Geometry: final body of the model. Coordinates: model frame, mm. A direction names the side the tool comes from. Give positions to 0.01 mm unless a question says otherwise; leave off trailing zeros. Write each loop counter-clockwise with the first axis right and the second up, starting at its lowest first coordinate (ties: lowest second). Pieces come first, ordered by that corner, then holes. Notation, with made-up numbers: M 47,64 L 63,64 A29 cw 63,88 Z; hole C 2.25,55.25 d5. An arc over 180 degrees is marked long. Use one line per item in the form item = value. Start each with the question number.
Item 1: Section query C-C on y = 55.5. Return loops of the section in (x, z).
Item 2: Material intervals for line 1 along Z through (x, y) = (-28.2, 8); line 2 along Y through (x, z) = (-15, -23); line 3 along X through (y, z) = (6, -28) (3 decimals), sorted ascending. Write a range as from..to.
Item 3: Section query D-D on z = -36. Return loops of the section in (x, y), then the cut area to 3 significant figures.
Item 4: Section query B-B on x = -18.5. Return loops of the section in (y, z), then the cut area to 3 significant figures.
Item 5: Contact query for flat-ended pins moving along their axis: P1, Ø5, axis at x = -29.5, y = 60, coming from the -Z side; P2, Ø10, axis at x = -8.5, z = -33, coming from the +Y side; P3, Ø8, axis at x = -24.5, y = 36, coming from the +Z side; P4, Ø3, axis at x = -30, z = -33, coming from the +Y side. Output: stop coordinate, or through.
Item 6: Pull-direction query (Z, two-part tool) for faces 5 (the flat face through (-28, 2, 0)), 6 (the cylindrical face through (-15.19, 25.71, -53.22)), 7 (the cylindrical face through (-24.385, 9.86, -26.999)); classes: released by +Z, released by -Z, zero draft, split by the parting line, or undercut.
Item 7: Section query A-A on y = 11. Return loops of the section in (x, z), then the cut area to 3 significant figures.
Item 8: Access query for faces 1 (the flat face through (-50, 5, -6)), 2 (the flat face through (-6, 5, -7)), 3 (the flat face through (-28, 53, -33)), 4 (the flat face through (-51, 5, -51)). Directions: +Z, -Z, +X, -X, +Y, -Y. A direction counts if a zero-diameter tool reaches every point of the face in a straight line with its end or side. Return the directions, or none.
Autodesk Inventor part; units mm, degrees
ref_plane "YZ Plane" through (0, 0, 0) normal (1, 0, 0) x (0, 1, 0)
ref_plane "XZ Plane" through (0, 0, 0) normal (0, 1, 0) x (-1, 0, 0)
ref_plane "XY Plane" through (0, 0, 0) normal (0, 0, 1) x (1, 0, 0)
sketch "Sketch1" plane through (0, 0, 0) normal (0, 1, 0) x (-1, 0, 0)
  line L0 (0, 0) -> (56.4, 0)
  line L1 (56.4, 0) -> (56.4, -56.4)
  line L2 (56.4, -56.4) -> (0, -56.4)
  line L3 (0, -56.4) -> (0, 0)
  dimension "d0" = 56.4
  dimension "d1" = 56.4
extrude "Extrusion1" add sketch "Sketch1" along normal blind 5
sketch "Sketch2" plane through (0, 5, 0) normal (0, 1, 0) x (1, 0, 0)
  circle A0 centre (-28.2, 28.2) radius 28.2
  line L0 (-56.4, 0) -> (0, 0)
  line L1 (-56.4, 56.4) -> (-56.4, 0)
  dimension "d4" = 56.4
  dimension "d5" = 28.2
  dimension "d6" = 28.2
extrude "Extrusion2" add sketch "Sketch2" along normal blind 42 contours A0
sketch "Sketch3" plane through (-28.2, 47, -28.2) normal (0, 1, 0) x (1, 0, 0)
  arc A0 (0, 28.2) -> (-28.2, 0) centre (0, 0) ccw
  circle A1 centre (0, 0) radius 6
  point P0 (28.2, -28.2)
  dimension "d9" = 12
extrude "g" add sketch "Sketch3" along normal blind 28
sketch "Sketch4" plane through (-28.2, 75, -28.2) normal (0, 1, 0) x (1, 0, 0)
  circle A0 centre (0, 0) radius 6
  line L0 (0, 0) -> (0, -6)
  line L1 (0, 0) -> (0, 3.5)
  line L2 (0, 3.5) -> (-5, 3.5)
  line L3 (0, 3.5) -> (5, 3.5)
  line L4 (5, 3.5) -> (-5, 3.5)
  line L5 (-5, 3.5) -> (-5, 8.5)
  line L6 (-5, 8.5) -> (5, 8.5)
  line L7 (5, 8.5) -> (5, 3.5)
  point P0 (28.2, -28.2)
  dimension "d12" = 3.5
  dimension "d13" = 5
  dimension "d14" = 5
  dimension "d15" = 10
  dimension "d16" = 5
extrude "Extrusion4" cut sketch "Sketch4" against normal blind 22 contours L2 L5 L6 L7 L3 A0 | A0 L3 L2
sketch "Sketch5" plane through (0, 0, 0) normal (0, -1, 0) x (1, 0, 0)
  circle A0 centre (-28.2, -28.2) radius 28.2
  circle A1 centre (-28.2, -28.2) radius 4
  point P0 (0, 0)
  dimension "d19" = 8
extrude "Extrusion5" cut sketch "Sketch5" against normal blind 20 contours A1
properties part number "2804S_NEMA2115_1Gearbox"
Answer sheet:
q1.outline = M -33.07,-31.7 L -23.33,-31.7 A6 ccw long Z
q2.line_1 = -56.4..-32.2, -24.2..0
q2.line_2 = 0..47
q2.line_3 = -56.399..-32.195, -24.205..-0.001
q3.outline = M -56.4,0 L 0,0 L 0,5 L -1.1,5 L -1.1,47 L -55.3,47 L -55.3,5 L -56.4,5 Z
q3.area = 2,560 mm2
q4.outline = M 0,-56.4 L 5,-56.4 L 5,-54.68 L 47,-54.68 L 47,-1.72 L 5,-1.72 L 5,0 L 0,0 Z
q4.area = 2,510 mm2
q5.P1 = -31.7
q5.P2 = 47
q5.P3 = 0
q5.P4 = 75
q6.face_5 = released by +Z
q6.face_6 = split by the parting line
q6.face_7 = undercut
q7.outline = C -28.2,-28.2 d56.4; hole C -28.2,-28.2 d8
q7.area = 2,450 mm2
q8.face_1 = +Z, -X, +Y
q8.face_2 = +Z, +X, +Y
q8.face_3 = -Z, +X, -X, +Y
q8.face_4 = -Z, -X, +Y
